```python
from build123d import *

# Parameters (mm, degrees)
F_1_8_0_125_CLEARANCE_DOWEL_HOLE1_D = 3.175
M3X0_5_TAPPED_HOLE2_D               = 2.5
M3X0_5_TAPPED_HOLE3_D               = 2.5
M3X0_5_TAPPED_HOLE3_DEPTH           = 7.5
M3X0_5_TAPPED_HOLE3_CSINK_D         = 3
M3X0_5_TAPPED_HOLE3_CSINK_ANGLE     = 90
M3X0_5_TAPPED_HOLE3_TIP             = 0.751075774
CHAMFER1_SIZE                       = 0.2
FILLET1_R                           = 1
FILLET2_R                           = 0.5


with BuildPart() as part:
    # Sketch1 → Revolve1 (revolve)
    with BuildSketch(Plane.XZ):
        Polygon((1.7, 11.75), (0, 11.75), (0, -73.5), (2.5, -73.5), (2.5, 0), (2, 0), (2, 0.75), (2.5, 0.75), (2.5, 10.364359355), align=None)
    revolve(axis=Axis((0, 0, 11.75), (0, 0, -1)))

    # 1/8 (0.125) Clearance Dowel Hole1 (through all)
    with Locations(Plane(origin=(0, -2.5, 7.75), x_dir=(-1, 0, 0), z_dir=(0, -1, 0))):
        with Locations((0, 0)):
            Hole(F_1_8_0_125_CLEARANCE_DOWEL_HOLE1_D / 2)

    # M3x0.5 Tapped Hole2 (through all)
    with Locations(Plane(origin=(-1.767766953, 1.767766953, -44), x_dir=(0.707106781, 0.707106781, 0), z_dir=(-0.707106781, 0.707106781, 0))):
        with Locations((0, 0)):
            Hole(M3X0_5_TAPPED_HOLE2_D / 2)

    # M3x0.5 Tapped Hole3
    with Locations(Plane(origin=(0, 0, -73.5), x_dir=(-1, 0, 0), z_dir=(0, 0, -1))):
        with Locations((0, 0)):
            CounterSinkHole(M3X0_5_TAPPED_HOLE3_D / 2, M3X0_5_TAPPED_HOLE3_CSINK_D / 2, depth=M3X0_5_TAPPED_HOLE3_DEPTH, counter_sink_angle=M3X0_5_TAPPED_HOLE3_CSINK_ANGLE)
            with Locations((0, 0, -(M3X0_5_TAPPED_HOLE3_DEPTH + M3X0_5_TAPPED_HOLE3_TIP / 2))):  # 118° drill point
                Cone(0, M3X0_5_TAPPED_HOLE3_D / 2, M3X0_5_TAPPED_HOLE3_TIP, mode=Mode.SUBTRACT)

    # Chamfer1
    chamfer1_edges = [part.edges().sort_by_distance(p)[0] for p in [
        (-2.5, 0, -73.5),
    ]]
    chamfer(chamfer1_edges, length=CHAMFER1_SIZE)

    # Fillet1
    fillet1_edges = [part.edges().sort_by_distance(p)[0] for p in [
        (-2.5, 0, 10.364359355),
    ]]
    fillet(fillet1_edges, radius=FILLET1_R)

    # Fillet2
    fillet2_edges = [part.edges().sort_by_distance(p)[0] for p in [
        (-1.7, 0, 11.75),
    ]]
    fillet(fillet2_edges, radius=FILLET2_R)


solid = part.part
```
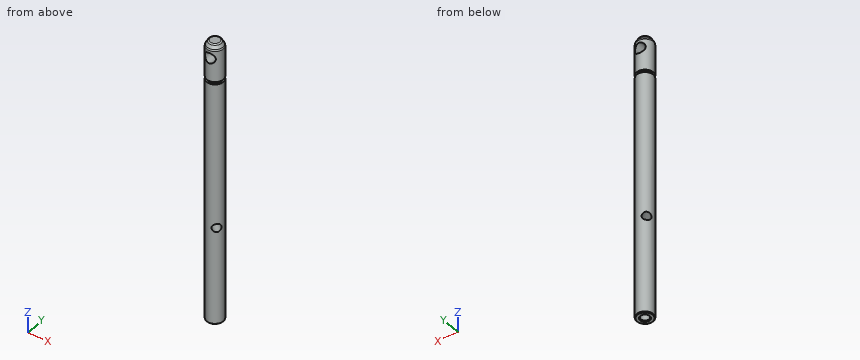
Source: CAD feature listing. Evaluate the final solid. Frame: model axes, mm. Give positions to 0.01 mm unless a question says otherwise; leave off trailing zeros. Write each loop counter-clockwise with the first axis right and the second up, starting at its lowest first coordinate (ties: lowest second). Pieces come first, ordered by that corner, then holes.
1. Material intervals for line 1 along Y through (x, z) = (0, -71); line 2 along X through (y, z) = (0.25, -19), sorted ascending.
2. Section query A-A (z = 7.75). Return the cut outline in (x, y), then the cut area to 3 significant figures.
3. Section query B-B (z = -58.5). Return the cut outline in (x, y).
4. First-contact query: pin 1 (3 mm diameter, centred on y = -1.5, z = 1, fed in from -X); pin 2 (1 mm diameter, centred on x = 1.5, z = -43, fed in from +Y); pin 3 (1.9 mm diameter, centred on x = 0, z = 7.75, fed in from -Y). Flat tips, straight axial feed; report the tip coordinate or a pass-through.
Output values:
1. line 1: y = -2.5 to -1.25, 1.25 to 2.5
1. line 2: x = -2.49 to 2.49
2. outline: (-1.59, -1.93) - (-1.59, 1.93) arc R2.5 ccw to start; (1.59, -1.93) arc R2.5 ccw to (1.59, 1.93) - close
2. area: 4.90 mm2
3. outline: circle Ø5 at (0, 0)
4. pin 1: stops at x = -2.5
4. pin 2: stops at y = 2.29
4. pin 3: passes through
